Source: CAD feature listing. Evaluate the final solid. Frame: model axes, mm. A direction names the side the tool comes from. Give positions to 0.01 mm unless a question says otherwise; leave off trailing zeros. Write each loop counter-clockwise with the first axis right and the second up, starting at its lowest first coordinate (ties: lowest second). Pieces come first, ordered by that corner, then holes. Notation, with made-up numbers: (41, -39.5) - (53, -39.5) arc R23 ccw to (53, -7.5) - close; hole circle Ø6 at (-6.75, -6.5). An arc over 180 degrees is marked (long way). Answer as a JSON object with one key per item and string values. Group by question number.
Autodesk Inventor part; units mm, degrees
ref_plane "Work Plane1" through (29, 0, 0) normal (0, -1, 0) x (1, 0, 0)
ref_plane "YZ Plane" through (0, 0, 0) normal (1, 0, 0) x (0, 1, 0)
ref_plane "XZ Plane" through (0, 0, 0) normal (0, 1, 0) x (-1, 0, 0)
sketch "Sketch1" plane through (0, 0, 0) normal (0, 0, 1) x (1, 0, 0)
  line L0 (-0.6667, 0) -> (18, 0)
  line L1 (18, 0) -> (18, 1.5)
  line L2 (18, 1.5) -> (3.3067, 1.5)
  line L3 (3.3067, 1.5) -> (2.9999, 1.5)
  line L4 (2.9999, 1.5) -> (0, 1.5)
  line L5 (0, 1.5) -> (0, 2.75)
  line L6 (0, 2.75) -> (-3, 2.75)
  line L7 (-3, 2.75) -> (-3, 1.4434)
  line L8 (-3, 1.4434) -> (-1.5, 1.4434)
  line L9 (-1.5, 1.4434) -> (-0.6667, 0)
  line L10 (-6.8, 0) -> (19.8, 0)
  line L11 (0, -0.55) -> (0, 3.3)
  line L12 (3.3067, 1.5) -> (0, 1.5) construction
  dimension "d1" = 14.6933
  dimension "d2" = 0.3068
  dimension "d3" = 3
  dimension "d4" = 1.5
  dimension "d5" = 60
  dimension "d6" = 3
  dimension "d7" = 3
  dimension "d8" = 2.8868
  dimension "d9" = 5.5
  dimension "d26" = 18
revolve "Body" add sketch "Sketch1" angle 360 about axis through (-0.6667, 0, 0) along (1, 0, 0)
sketch "Sketch2" plane through (-3, 0, 0) normal (-1, 0, 0) x (0, 0, 1)
  circle A0 centre (0, 0) radius 1.4434
  line L0 (0, -3.85) -> (0, 3.85)
  line L1 (-3.85, 0) -> (3.85, 0)
  line L2 (1.4434, 0) -> (0.7217, -1.25)
  line L3 (0.7217, -1.25) -> (-0.7217, -1.25)
  line L4 (-0.7217, -1.25) -> (-1.4434, 0)
  line L5 (-1.4434, 0) -> (-0.7217, 1.25)
  line L6 (-0.7217, 1.25) -> (0.7217, 1.25)
  line L7 (0.7217, 1.25) -> (1.4434, 0)
extrude "Slot" add sketch "Sketch2" against normal up to next contours L7 A0 | A0 L2 | L6 L0 A0 | A0 L0 L3 | L0 L6 A0 | A0 L3 L0 | L4 A0 | A0 L5
fillet "Fillet1" radius 0.3 1 edges at (-3, -2.75, 0)
thread "Thread"
chamfer "Chamfer1" distance 0.3067 distance2 0.3067 1 edges at (18, -1.5, 0) measured on face at (18, -0.4645, -0.4115)
ref_plane "Work Plane1" through (29, 0, 0) normal (0, -1, 0) x (1, 0, 0)
fillet "Fillet2" radius 0.1 1 edges at (0, -1.5, 0)
equation "\"d1\" = GEL"
equation "\"d3\" = KOH"
equation "\"d4\" = INTI"
equation "\"d6\" = GD"
equation "\"d7\" = BDM"
equation "\"d8\" = 1.1547 * SW"
equation "\"d9\" = KOD"
equation "\"d26\" = NLG"
equation "\"d30\" = R"
equation "\"d17\" = RR"
equation "\"d13\" = GEL"
equation "\"d15\" = -0.5 * SPD + 0.5 * GD"
equation "\"d16\" = GUL"
equation "\"GD\" = NND"
equation "\"NLG\" = 18"
equation "\"GEL\" = 14.69328"
equation "\"KOD\" = 5.5"
equation "\"KOH\" = 3"
equation "\"INTI\" = 1.5"
equation "\"GAL\" = 0.61345 * PTC"
equation "\"GUL\" = 0.61345 * PTC"
equation "\"BDM\" = NND"
equation "\"SW\" = 2.5"
equation "\"RR\" = 0.3"
equation "\"SPD\" = 2.38655"
equation "\"R\" = 0.1"
equation "\"TOA\" = 30deg"
equation "\"THREADDIA\" = 3"
equation "\"PTC\" = 0.5"
equation "\"NND\" = 3"
equation "\"E0\" = 1.155 * SW"
equation "\"GD1\" = THREADDIA - 1.2269 * PTC"
properties part number "M3x18" material "Steel, Mild"
Q1. Draft query along Z for faces 4 (the cylindrical face through (-1.369, -0.596, 2.685)), 5 (the flat face through (18, 0, 0)), 6 (the flat face through (-2.205, 0.616, -1.088)). Return one class per face: released by +Z, released by -Z, zero draft, split by the parting line, or undercut.
Q2. Ray query, probe 1 along X at (y, z) = (1.95, 0.7); probe 2 along Y at (x, z) = (6, -0.05); probe 3 along X at (y, z) = (1.4, 0.15). Return the intervals inside material, ascending. Write a range as [from, to].
Q3. Reachability of faces 1 (the flat face through (0, 2, 0)), 2 (the flat face through (-3, -1.1, 1.1)), 3 (the flat face through (-2.21, 0.63, 1.08)) from +Z, -Z, +X, -X, +Y, -Y: full face, straight path, thin tool, end or side. Return the list, or none.
Q4. First-contact query: pin 1 Ø3 at (x, z) = (14, -1.5) entering from -Y; pin 2 Ø1 at (x, y) = (12.5, -1.5) entering from -Z. Flat tips, straight axial feed; report the tip coordinate or a pass-through.
Q5. Section A-A on x = 5. Return the cut outline in (y, z).
Taken from the geometry:
{
 "1": {"face 4": "split by the parting line", "face 5": "zero draft", "face 6": "undercut"},
 "2": {"probe 1": "x = [-3, 0]", "probe 2": "y = [-1.5, 1.5]", "probe 3": "x = [-3, 17.79]"},
 "3": {"face 1": "+X", "face 2": "+Z, -Z, -X, +Y, -Y", "face 3": "-X"},
 "4": {"pin 1": "stops at y = -1.5", "pin 2": "stops at z = -1.12"},
 "5": {"outline": "circle Ø3 at (0, 0)"}
}
